Read the model definition and answer for the solid it produces. Units are mm, in the model's axes. A direction names the side the tool comes from. Coordinates: 2 decimals unless noted, no trailing zeros. Loops run counter-clockwise (first coordinate to the right, second up) from the corner with the lowest first, then second, coordinate; pieces in that order, holes last.
Q1. Which of the six approach directions +Z, -Z, +X, -X, +Y, -Y give full straight-line access (tool end or side, diameter ignored) to faces 5 (the face through (2.24, 0.05, 19.14)), 6 (the face through (-3, 0, 0)), 7 (the face through (-0.33, 2.52, 6.44))?
Q2. Section B-B (x = 0) is taken. Give the vertices of the cut face in (y, z).
Q3. The mould has two halves that part along X. Classify faces 1 (the face through (-13.737, 0.113, 6.261)), 2 (the face through (-8, 0, 6.35)), 3 (the face through (0, 2, 25.4)), 4 (the face through (13.737, -0.113, 6.261)): pulls with the +X half, pulls with the -X half, needs draft (parallel to the pull), parting line crosses it, or undercut.
Q4. Section D-D (x = 7.62) is taken. Give the vertices of the cut face in (y, z), then the cut area to 3 significant figures.
Q5. Straight lines are drawn through the part: line 1 (Y direction, x = -7.5, z = 5.75); line 2 (Y direction, x = 0, z = 8.25); line 3 (Z direction, x = -4, y = -7). For each, find the intervals that lie inside material, in ascending order.
Q6. Section C-C (z = 4.75) is taken. Give the vertices of the cut face in (x, y), then the cut area to 3 significant figures.
Q7. Section A-A (y = 0) is taken. Count the separate pieces of the cut face and the enclosed holes in it, then the cut area to 3 significant figures.
Q8. Flat-ended cylindrical pins translate along their axes: P1, Ø4.5, axis at x = 7.62, y = 0, coming from the -Z side; P2, Ø5, axis at y = 4.5, z = 9, coming from the +X side; P3, Ø1.5, axis at x = -1.5, z = 17, coming from the +Y side. Find the tip coordinate at first contact, or state that the pin passes through.
from build123d import *

# Parameters (mm, degrees)
F1_DEPTH = 12.7
F2_R     = 2.54
F3_DEPTH = 12.701
F4_R     = 6.35
F5_DEPTH = 12.7
F6_R     = 2.38125
F7_DEPTH = 6.35
F8_R     = 1.190625
F9_DEPTH = 12.7


with BuildPart() as f1:
    # F0 (on Top) → F1 (new body)
    with BuildSketch(Plane.XY):
        with BuildLine():
            Line((-11.43, -7.62), (11.43, -7.62))
            ThreePointArc((11.43, -7.62), (13.73715, 0), (11.43, 7.62))
            Line((11.43, 7.62), (-11.43, 7.62))
            ThreePointArc((-11.43, 7.62), (-13.73715, 0), (-11.43, -7.62))
        make_face()
    extrude(amount=F1_DEPTH)

    # F2 (on face) → F3 (cut, through all)
    with BuildSketch(Plane.XY.offset(12.7)):
        Circle(F2_R)
    extrude(amount=-F3_DEPTH, mode=Mode.SUBTRACT)

    # F4 (on face) → F5 (join)
    with BuildSketch(Plane.XY.offset(12.7)):
        Circle(F4_R)
    extrude(amount=F5_DEPTH)

    # F6 (on face) → F7 (cut)
    with BuildSketch(Plane(origin=(0, 0, 0), x_dir=(1, 0, 0), z_dir=(0, 0, -1))):
        with Locations((-7.62, 0)):
            Circle(F6_R)
        with Locations((7.62, 0)):
            Circle(F6_R)
    extrude(amount=-F7_DEPTH, mode=Mode.SUBTRACT)

    # F8 (on face) → F9 (cut)
    with BuildSketch(Plane.XY.offset(25.4)):
        with Locations((-3.429, 0)):
            Circle(F8_R)
        with Locations((3.429, 0)):
            Circle(F8_R)
        Circle(F8_R)
    extrude(amount=-F9_DEPTH, mode=Mode.SUBTRACT)


solid = f1.part
Numbers:
1. face 5: +Z
1. face 6: -Z, +X, -X, +Y, -Y
1. face 7: -Z
2. outline: (-7.62, 0) - (-2.54, 0) - (-2.54, 12.7) - (-1.19, 12.7) - (-1.19, 25.4) - (-6.35, 25.4) - (-6.35, 12.7) - (-7.62, 12.7) - close; (1.19, 12.7) - (2.54, 12.7) - (2.54, 0) - (7.62, 0) - (7.62, 12.7) - (6.35, 12.7) - (6.35, 25.4) - (1.19, 25.4) - close
3. face 1: pulls with the -X half
3. face 2: undercut
3. face 3: needs draft
3. face 4: pulls with the +X half
4. outline: (-7.62, 0) - (-2.38, 0) - (-2.38, 6.35) - (2.38, 6.35) - (2.38, 0) - (7.62, 0) - (7.62, 12.7) - (-7.62, 12.7) - close
4. area: 163 mm2
5. line 1: y = -7.62 to -2.38, 2.38 to 7.62
5. line 2: y = -7.62 to -2.54, 2.54 to 7.62
5. line 3: z = 0 to 12.7
6. outline: (-11.43, -7.62) - (11.43, -7.62) arc R13.74 ccw to (11.43, 7.62) - (-11.43, 7.62) arc R13.74 ccw to start; hole circle Ø4.76 at (-7.62, 0); hole circle Ø5.08 at (0, 0); hole circle Ø4.76 at (7.62, 0)
6. area: 340 mm2
7. separate pieces: 4
7. enclosed holes: 0
7. area: 294 mm2
8. P1: stops at z = 6.35
8. P2: stops at x = 13.59
8. P3: stops at y = 6.31
